Input: part model. Units: mm. Frame: model coordinates. A direction names the side the tool comes from. Give positions to 0.01 mm unless a question says otherwise; leave off trailing zeros. Loops run counter-clockwise (first coordinate to the right, second up) from the corner with the lowest first, then second, coordinate; pieces in that order, holes last. Notation, with made-up numbers: M 78.25,10 L 127.25,10 A25 ccw 127.25,49 Z; hole C 79,48 d11. An arc over 180 degrees is marked long. One line per item, written item: value. Start each with the question number.
(1) Pin query (flat end, axial travel): P1, Ø1, axis at x = -1, y = -1, coming from the -Z side; P2, Ø1, axis at y = -1.5, z = 1, coming from the +X side. Return the tip coordinate at first contact, or that it passes through.
(2) Ray query, line 1 along X through (y, z) = (-1.35, 71); line 2 along Z through (x, y) = (-0.25, -1.6); line 3 along Z through (x, y) = (9.5, -0.8). Return the intervals inside material, ascending. Write a range as from..to.
(3) Section B-B on x = 7.5. Output: boundary loops of the cut face in (y, z), plus the area to 3 significant figures.
(4) Section C-C on y = -0.4. Output: boundary loops of the cut face in (x, z), plus the area to 3 significant figures.
(5) Access query for faces 1 (the cylindrical face through (7.4, -1, 97)), 2 (the flat face through (15, -1, 1)), 3 (the flat face through (8, -1, 102)). Directions: +Z, -Z, +X, -X, +Y, -Y. A direction counts if a zero-diameter tool reaches every point of the face in a straight line with its end or side. Return the directions, or none.
(6) Pull-direction query (X, two-part tool) for faces 4 (the flat face through (4.5, -1, 69)), 5 (the flat face through (-1, -1, 2)), 6 (the flat face through (0, -1, 1)); classes: released by +X, released by -X, zero draft, split by the parting line, or undercut.
(7) Section A-A on z = 62. Output: boundary loops of the cut face in (x, y), plus the area to 3 significant figures.
```python
from build123d import *

# Parameters (mm, degrees)
F1_DEPTH = 2


with BuildPart() as f1:
    # F0 (on Front) → F1 (new body)
    with BuildSketch(Plane.XZ):
        Polygon((0, 2), (0, 0), (15, 0), (15, 2), (17.5, 2), (17.5, 102), (-2.5, 102), (-2.5, 2), align=None)
        with BuildLine():
            Line((4.5, 44), (4.5, 94))
            ThreePointArc((4.5, 94), (7.5, 97), (10.5, 94))
            Line((10.5, 94), (10.5, 44))
            ThreePointArc((10.5, 44), (7.5, 41), (4.5, 44))
        make_face(mode=Mode.SUBTRACT)
    extrude(amount=F1_DEPTH)


solid = f1.part
```
Output values:
1. P1: stops at z = 2
1. P2: stops at x = 15
2. line 1: x = -2.5..4.5, 10.5..17.5
2. line 2: z = 2..102
2. line 3: z = 0..41.76, 96.24..102
3. outline: M -2,0 L 0,0 L 0,41 L -2,41 Z; M -2,97 L 0,97 L 0,102 L -2,102 Z
3. area: 92.0 mm²
4. outline: M -2.5,2 L 0,2 L 0,0 L 15,0 L 15,2 L 17.5,2 L 17.5,102 L -2.5,102 Z; hole M 4.5,44 A3 ccw 10.5,44 L 10.5,94 A3 ccw 4.5,94 Z
4. area: 1,700 mm²
5. face 1: +Y, -Y
5. face 2: -Z, +X, +Y, -Y
5. face 3: +Z, +X, -X, +Y, -Y
6. face 4: undercut
6. face 5: zero draft
6. face 6: released by -X
7. outline: M -2.5,-2 L 4.5,-2 L 4.5,0 L -2.5,0 Z; M 10.5,-2 L 17.5,-2 L 17.5,0 L 10.5,0 Z
7. area: 28.0 mm²
